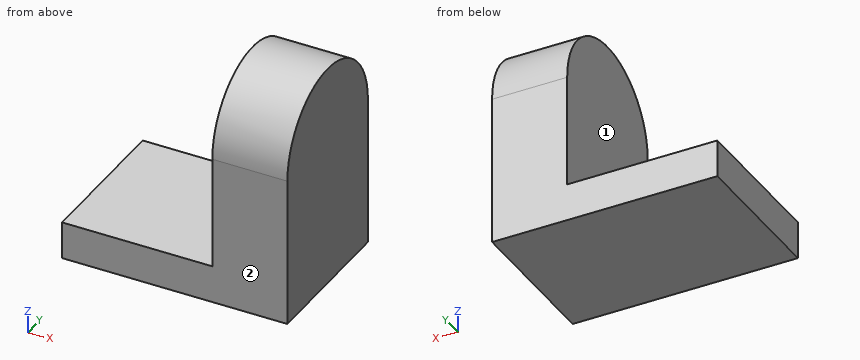
from build123d import *

# Parameters (mm, degrees)
F1_DEPTH = 38.1
F2_W     = 106.504818
F2_H     = 101.6
F3_DEPTH = 25.4


with BuildPart() as f1:
    # F0 (on Right) → F1 (new body)
    with BuildSketch(Plane.YZ):
        with BuildLine():
            Line((0, 25.4), (0, 0))
            Line((0, 0), (25.4, 0))
            Line((25.4, 0), (25.4, 25.4))
            ThreePointArc((25.4, 25.4), (12.7, 38.1), (0, 25.4))
        make_face()
    extrude(amount=F1_DEPTH)

    # F2 (on Right) → F3 (cut)
    with BuildSketch(Plane.YZ):
        with Locations((53.252409, 57.15)):
            Rectangle(F2_W, F2_H)
    extrude(amount=F3_DEPTH, mode=Mode.SUBTRACT)


solid = f1.part
Check sheet for the modelled part. Datum: model origin and axes. Units: mm. Face numbers are marked on the shaded views. A direction names the side the tool comes from. Coordinates: 2 decimals unless noted, no trailing zeros. Loops run counter-clockwise (first coordinate to the right, second up) from the corner with the lowest first, then second, coordinate; pieces in that order, holes last. Notation, with made-up numbers: (12.5, 89.25) -> (16.5, 89.25) arc R28 ccw to (16.5, 119.25) -> close; hole circle Ø11 at (68, -8.75). An arc over 180 degrees is marked (long way). Write item = value, one per line. Start each with the question number.
1. Tool access check on the marked faces 1 and 2. Record the directions out of +Z, -Z, +X, -X, +Y, -Y that give a thin tool (end or side, any length) a straight path to the whole face; none if there is none.
2. Section check A-A on x = 30. Record the cut outline in (y, z).
3. Section check C-C on z = 12. Record the cut outline in (x, y), then the cut area to 3 significant figures.
4. Section check D-D on y = 6.5. Record the cut outline in (x, z), then the cut area to 3 significant figures.
5. Material ranges on line 1 (X direction, y = 6, z = 33.5); line 2 (Z direction, x = 11, y = 21.5); line 3 (Z direction, x = 26.5, y = 13), recorded low to high.
6. Section check B-B on y = 13.75. Record the cut outline in (x, z).
7. Depth check by flat-ended pin: P1, Ø12.5, axis at x = 16.5, y = 9.5, coming from the +Z side. Enter the tip coordinate at first touch or a pass-through.
Responses:
q1.face_1 = +Z, -X, +Y, -Y
q1.face_2 = +Z, -Z, +X, -X, -Y
q2.outline = (0, 0) -> (25.4, 0) -> (25.4, 25.4) arc R12.7 ccw to (0, 25.4) -> close
q3.outline = (25.4, 0) -> (38.1, 0) -> (38.1, 25.4) -> (25.4, 25.4) -> close
q3.area = 323 mm2
q4.outline = (0, 0) -> (38.1, 0) -> (38.1, 36.48) -> (25.4, 36.48) -> (25.4, 6.35) -> (0, 6.35) -> close
q4.area = 625 mm2
q5.line_1 = 25.4 to 38.1
q5.line_2 = 0 to 6.35
q5.line_3 = 0 to 38.1
q6.outline = (0, 0) -> (38.1, 0) -> (38.1, 38.06) -> (25.4, 38.06) -> (25.4, 6.35) -> (0, 6.35) -> close
q7.P1 = 6.35
